Build history of the part. All positions in model axes, mm. A direction names the side the tool comes from. Coordinates: 2 decimals unless noted, no trailing zeros. Loops run counter-clockwise (first coordinate to the right, second up) from the corner with the lowest first, then second, coordinate; pieces in that order, holes last.
Item 1: Flat gauge pins, fed straight in: pin 1 (4 mm diameter, centred on x = -29, y = 4, fed in from -Z); pin 2 (5 mm diameter, centred on x = 32.25, y = 0, fed in from +Z). Where does each tip first touch, or does it go through?
Item 2: Cut at D-D (x = -20). List the corners of the cut face in (y, z), and give its area (3 significant figures).
Item 3: 3-axis set-ups, long thin cutter, end or side, ignore diameter. For faces 4 (the face through (35, -4, 2)), 5 (the face through (35, 4, 2)), 6 (the face through (-1, 0, 0)): which of +Z, -Z, +X, -X, +Y, -Y reach the whole face in a straight line?
Item 4: Cut at C-C (z = 2.15). List the corners of the cut face in (x, y) (3 decimals).
Item 5: Mould opens along Z. For faces 1 (the face through (0, 4, 3)), 2 (the face through (-38.25, 0, 3)), 3 (the face through (-1, 0, 6)) say: released by +Z, released by -Z, zero draft, split by the parting line, or undercut.
Item 6: Cut at B-B (x = 32.25). List the corners of the cut face in (y, z), and give its area (3 significant figures).
Item 7: Cut at A-A (y = 0). List the corners of the cut face in (x, z), and give its area (3 significant figures).
Item 8: Drill centre lines: line 1 along X through (y, z) = (0, 3.75); line 2 along Y through (x, z) = (32.25, 3.5); line 3 along X through (y, z) = (-2.75, 0.3). Where is each one in solid material? Low to high.
from build123d import *

# Parameters (mm, degrees)
SKETCH_1_W          = 70
SKETCH_1_H          = 10
EXTRUDE_1_DEPTH     = 6
SKETCH_2_W          = 1.5
SKETCH_2_H          = 1.5
CUT_EXTRUDE_1_DEPTH = 71.434366612
SKETCH_3_R          = 3
CUT_EXTRUDE_2_DEPTH = 36.860842154
SKETCH_4_R          = 3
CUT_EXTRUDE_3_DEPTH = 36.860842154
SKETCH_5_W          = 3.25
SKETCH_5_H          = 10
EXTRUDE_2_DEPTH     = 6
SKETCH_9_R          = 3
CUT_EXTRUDE_4_DEPTH = 40.039243077
SKETCH_10_R         = 3
EXTRUDE_4_DEPTH     = 6
SKETCH_11_R         = 3
CUT_EXTRUDE_5_DEPTH = 40.039243077


with BuildPart() as part:
    # 草图1 → 凸台-拉伸1 (new body)
    with BuildSketch(Plane.XY):
        Rectangle(SKETCH_1_W, SKETCH_1_H)
    extrude(amount=EXTRUDE_1_DEPTH)

    # 草图2 → 切除-拉伸1 (cut, through all)
    with BuildSketch(Plane.ZY.offset(35)):
        with Locations((2.25, 4.25)):
            Rectangle(SKETCH_2_W, SKETCH_2_H)
        with Locations((2.25, -4.25)):
            Rectangle(SKETCH_2_W, SKETCH_2_H)
    extrude(amount=-CUT_EXTRUDE_1_DEPTH, mode=Mode.SUBTRACT)

    # 草图3 → 切除-拉伸2 (cut, through all)
    with BuildSketch(Plane.XY.offset(6)):
        with Locations((-29, 0)):
            Circle(SKETCH_3_R)
        with Locations((29, 0)):
            Circle(SKETCH_3_R)
    extrude(amount=-CUT_EXTRUDE_2_DEPTH, mode=Mode.SUBTRACT)

    # 草图4 → 切除-拉伸3 (cut, through all)
    with BuildSketch(Plane.XY.offset(6)):
        with Locations((-32.25, 0)):
            Circle(SKETCH_4_R)
    extrude(amount=-CUT_EXTRUDE_3_DEPTH, mode=Mode.SUBTRACT)

    # 草图5 → 凸台-拉伸2 (add)
    with BuildSketch(Plane.XY.offset(6)):
        with Locations((36.625, 0)):
            Rectangle(SKETCH_5_W, SKETCH_5_H)
        with Locations((-36.625, 0)):
            Rectangle(SKETCH_5_W, SKETCH_5_H)
    extrude(amount=-EXTRUDE_2_DEPTH)

    # 草图9 → 切除-拉伸4 (cut, through all)
    with BuildSketch(Plane.XY.offset(6)):
        with BuildLine():
            ThreePointArc((-30.625, -2.521780125), (-32, 0), (-30.625, 2.521780125))
            ThreePointArc((-30.625, 2.521780125), (-33.118257406, 2.871607403), (-35, 1.198957881))
            Line((-35, 1.198957881), (-35, -1.198957881))
            ThreePointArc((-35, -1.198957881), (-33.118257406, -2.871607403), (-30.625, -2.521780125))
        make_face()
        with BuildLine():
            Line((-35, -1.198957881), (-35, 1.198957881))
            ThreePointArc((-35, 1.198957881), (-35.25, 0), (-35, -1.198957881))
        make_face()
        with Locations((-29, 0)):
            Circle(SKETCH_9_R)
        with Locations((-32.25, 0)):
            Circle(SKETCH_9_R)
        with Locations((32.25, 0)):
            Circle(SKETCH_9_R)
        with Locations((29, 0)):
            Circle(SKETCH_9_R)
    extrude(amount=-CUT_EXTRUDE_4_DEPTH, mode=Mode.SUBTRACT)

    # 草图10 → 凸台-拉伸4 (add)
    with BuildSketch(Plane.XY.offset(6)):
        with Locations((-29, 0)):
            Circle(SKETCH_10_R)
        with Locations((29, 0)):
            Circle(SKETCH_10_R)
    extrude(amount=-EXTRUDE_4_DEPTH)

    # 草图11 → 切除-拉伸5 (cut, through all)
    with BuildSketch(Plane.XY.offset(6)):
        with Locations((-32.25, 0)):
            Circle(SKETCH_11_R)
        with Locations((32.25, 0)):
            Circle(SKETCH_11_R)
    extrude(amount=-CUT_EXTRUDE_5_DEPTH, mode=Mode.SUBTRACT)


solid = part.part
Filled sheet:
1. pin 1: stops at z = 0
1. pin 2: passes through
2. outline: (-5, 0) - (5, 0) - (5, 1.5) - (3.5, 1.5) - (3.5, 3) - (5, 3) - (5, 6) - (-5, 6) - (-5, 3) - (-3.5, 3) - (-3.5, 1.5) - (-5, 1.5) - close
2. area: 55.5 mm2
3. face 4: -Y
3. face 5: +Y
3. face 6: -Z, +X, -X, +Y, -Y
4. outline: (-38.25, -5) - (-35, -5) - (-35, -3.5) - (35, -3.5) - (35, -5) - (38.25, -5) - (38.25, 5) - (35, 5) - (35, 3.5) - (-35, 3.5) - (-35, 5) - (-38.25, 5) - close; hole circle Ø6 at (-32.25, 0); hole circle Ø6 at (32.25, 0)
5. face 1: undercut
5. face 2: zero draft
5. face 3: released by +Z
6. outline: (-5, 0) - (-3, 0) - (-3, 6) - (-5, 6) - (-5, 3) - (-3.5, 3) - (-3.5, 1.5) - (-5, 1.5) - close; (3, 0) - (5, 0) - (5, 1.5) - (3.5, 1.5) - (3.5, 3) - (5, 3) - (5, 6) - (3, 6) - close
6. area: 19.5 mm2
7. outline: (-38.25, 0) - (-35.25, 0) - (-35.25, 6) - (-38.25, 6) - close; (-29.25, 0) - (29.25, 0) - (29.25, 6) - (-29.25, 6) - close; (35.25, 0) - (38.25, 0) - (38.25, 6) - (35.25, 6) - close
7. area: 387 mm2
8. line 1: x = -38.25 to -35.25, -29.25 to 29.25, 35.25 to 38.25
8. line 2: y = -5 to -3, 3 to 5
8. line 3: x = -38.25 to -33.45, -31.05 to 31.05, 33.45 to 38.25
